Build history of the part. All positions in model axes, mm. A direction names the side the tool comes from. Give positions to 0.01 mm unless a question says otherwise; leave off trailing zeros. Write each loop counter-clockwise with the first axis right and the second up, starting at its lowest first coordinate (ties: lowest second). Pieces come first, ordered by that corner, then holes. Notation, with made-up numbers: (59, -12.5) -> (68, -12.5) arc R22 ccw to (68, 25.5) -> close; hole circle Ø10 at (23, 16.25). An arc over 180 degrees is marked (long way). Put each result on its own line as item: value. Start each with the question number.
Item 1: Slice it at B-B, the plane y = 0.5. List the corners of the cut face in (x, z), plus the area to 3 significant figures.
Item 2: Slice it at C-C, the plane x = -1.5. List the corners of the cut face in (y, z).
Item 3: Tool access for faces 5 (the flat face through (-8.5, 0, 8)), 6 (the flat face through (10.5, 0, 7)): list every direction of +Z, -Z, +X, -X, +Y, -Y with a clear straight run to the whole face (end or side of a thin tool).
Item 4: Slice it at A-A, the plane z = 11. List the corners of the cut face in (x, y).
Item 5: Drill centre lines: line 1 along X through (y, z) = (0.15, 11); line 2 along Y through (x, z) = (1.75, 10); line 3 along Z through (x, y) = (6.5, -0.4). Where is each one in solid material? Low to high.
Item 6: Two-plate mould, pull along Y, no slides. Class faces 1 (the cylindrical face through (0.13, -2.07, 0.45)), 2 (the flat face through (0, 0, 3)), 3 (the flat face through (0, 2.5, 7)), 4 (the flat face through (0, 0, 0)): pulls with the +Y half, pulls with the -Y half, needs draft (parallel to the pull), parting line crosses it, or undercut.
```python
from build123d import *

# Parameters (mm, degrees)
SKETCH_W     = 21
SKETCH_H     = 5
PAD_DEPTH    = 13
SKETCH001_W  = 17
SKETCH001_H  = 2
POCKET_DEPTH = 10
FILLET_R     = 1.5
FILLET001_R  = 1


with BuildPart() as part:
    # Sketch → Pad (new body)
    with BuildSketch(Plane.XY):
        Rectangle(SKETCH_W, SKETCH_H)
    extrude(amount=PAD_DEPTH)

    # Sketch001 (on Face6 of Pad) → Pocket (cut)
    with BuildSketch(Plane.XY.offset(13)):
        Rectangle(SKETCH001_W, SKETCH001_H)
    extrude(amount=-POCKET_DEPTH, mode=Mode.SUBTRACT)

    # Fillet
    fillet_edges = [part.edges().sort_by_distance(p)[0] for p in [
        (0, 2.5, 0),
        (0, -2.5, 0),
        (10.5, 0, 0),
        (-10.5, 0, 0),
    ]]
    fillet(fillet_edges, radius=FILLET_R)

    # Fillet001
    fillet001_edges = [part.edges().sort_by_distance(p)[0] for p in [
        (-10.5, 2.5, 7.25),
        (-10.5, -2.5, 7.25),
        (10.5, 2.5, 7.25),
        (10.5, -2.5, 7.25),
    ]]
    fillet(fillet001_edges, radius=FILLET001_R)


solid = part.part
```
Values follow:
1. outline: (-10.5, 1.5) arc R1.5 ccw to (-9, 0) -> (9, 0) arc R1.5 ccw to (10.5, 1.5) -> (10.5, 13) -> (8.5, 13) -> (8.5, 3) -> (-8.5, 3) -> (-8.5, 13) -> (-10.5, 13) -> close
1. area: 102 mm2
2. outline: (-2.5, 1.5) arc R1.5 ccw to (-1, 0) -> (1, 0) arc R1.5 ccw to (2.5, 1.5) -> (2.5, 13) -> (1, 13) -> (1, 3) -> (-1, 3) -> (-1, 13) -> (-2.5, 13) -> close
3. face 5: +Z
3. face 6: +Z, -Z, +X, +Y, -Y
4. outline: (-10.5, -1.5) arc R1 ccw to (-9.5, -2.5) -> (9.5, -2.5) arc R1 ccw to (10.5, -1.5) -> (10.5, 1.5) arc R1 ccw to (9.5, 2.5) -> (-9.5, 2.5) arc R1 ccw to (-10.5, 1.5) -> close; hole (-8.5, -1) -> (8.5, -1) -> (8.5, 1) -> (-8.5, 1) -> close
5. line 1: -10.5 to -8.5, 8.5 to 10.5
5. line 2: -2.5 to -1, 1 to 2.5
5. line 3: 0 to 3
6. face 1: pulls with the -Y half
6. face 2: undercut
6. face 3: pulls with the +Y half
6. face 4: needs draft
